The listing builds one solid part. Answer for the finished solid, in the listing's coordinates (mm). Give positions to 0.01 mm unless a question says otherwise; leave off trailing zeros. Order: outer loops, then holes, each group sorted by start corner. A loop starts at its lowest first (then second) coordinate and runs counter-clockwise, first axis right, second up. Notation, with made-up numbers: (-8, 30) - (6, 30) arc R32 ccw to (6, 69) - close; hole circle Ø2 at (-36.75, -5.75). An arc over 180 degrees is marked (long way). Use a Markdown table: item, result. Add a question column.
1) Find section A-A, the plane y = 0.2. Determine the outline of the cut face in (x, z), plus the area to 3 significant figures.
2) Find section C-C, the plane x = 22. Determine the outline of the cut face in (y, z).
3) Find section B-B, the plane z = 154. Determine the outline of the cut face in (x, y).
4) Straight lines are drawn through the part: line 1 (X direction, y = -0.5, z = 107.5); line 2 (Z direction, x = 21.5, y = 0.95); line 3 (Z direction, x = 25, y = -0.4). For each, find the intervals that lie inside material, in ascending order.
5) A flat-ended cylindrical pin translates along its axis: pin 1 (1.2 mm diameter, centred on y = 0.5, z = 173, fed in from +X). Find the tip coordinate at first contact, or state that the pin passes through.
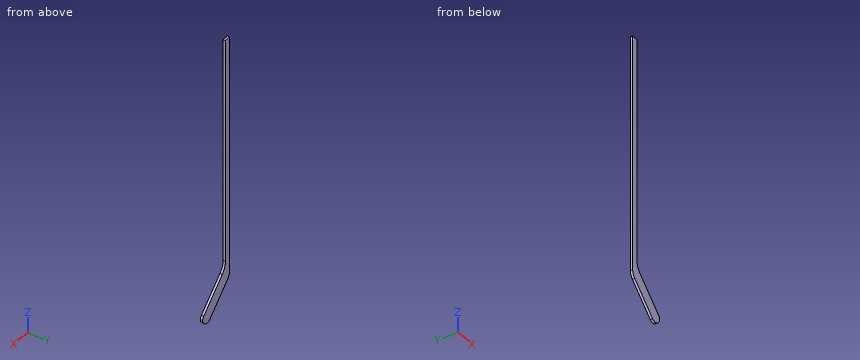
from build123d import *

# Parameters (mm, degrees)
F1_DEPTH = 1.15
F2_R     = 5
F3_R     = 10
F5_R     = 15


with BuildPart() as f1:
    # F0 (on Front) → F1 (new body, symmetric)
    with BuildSketch(Plane.XZ):
        Polygon((0, 240), (0, 0), (31.8198051534, -31.8198051534), (40.3050865276, -23.3345237792), (6, 10.9705627485), (6, 240), align=None)
    extrude(amount=F1_DEPTH, both=True)

    # F2
    f2_edges = [f1.edges().sort_by_distance(p)[0] for p in [
        (31.819805, 0, -31.819805),
        (40.305087, 0, -23.334524),
    ]]
    fillet(f2_edges, radius=F2_R)

    # F3
    f3_edges = [f1.edges().sort_by_distance(p)[0] for p in [
        (0, 0, 0),
    ]]
    fillet(f3_edges, radius=F3_R)

    # F5
    f5_edges = [f1.edges().sort_by_distance(p)[0] for p in [
        (6, 0, 10.970563),
    ]]
    fillet(f5_edges, radius=F5_R)


solid = f1.part
The answers:
| question | item | result |
|---|---|---|
| 1 | outline | (0, 4.14) arc R10 ccw to (2.93, -2.93) - (28.28, -28.28) arc R5 ccw to (35.36, -28.28) - (36.77, -26.87) arc R5 ccw to (36.77, -19.8) - (10.39, 6.58) arc R15 cw to (6, 17.18) - (6, 240) - (0, 240) - close |
| 1 | area | 1,960 mm2 |
| 2 | outline | (-1.15, -22) - (1.15, -22) - (1.15, -5.03) - (-1.15, -5.03) - close |
| 3 | outline | (0, -1.15) - (6, -1.15) - (6, 1.15) - (0, 1.15) - close |
| 4 | line 1 | 0 to 6 |
| 4 | line 2 | -21.5 to -4.53 |
| 4 | line 3 | -25 to -8.03 |
| 5 | pin 1 | x = 6 |
